For this review, take the finished solid that the model builds, in its own axes (mm). A direction names the side the tool comes from. Round coordinates to 2 decimals unless told otherwise and drop trailing zeros. Order: outer loops, then holes, each group sorted by start corner. A loop starts at its lowest first (then second) coordinate and runs counter-clockwise, first axis right, second up. Notation, with made-up numbers: (13.25, 20.25) - (32.25, 20.25) arc R27 cw to (32.25, 48.25) - close; hole circle Ø9 at (16, -27). An arc over 180 degrees is marked (long way). One line per question, with ' | ' between items.
```python
from build123d import *

# Parameters (mm, degrees)
ESQUISSE1_W                             = 30
ESQUISSE1_H                             = 10
BOSS_EXTRU_1_DEPTH                      = 130.5
ESQUISSE2_W                             = 30
ESQUISSE2_H                             = 5
BOSS_EXTRU_2_DEPTH                      = 20
PER_AGE_POUR_CROUS_AUTO_BLOQUANTS_300_D = 4.7625


with BuildPart() as part:
    # Esquisse1 → Boss.-Extru.1 (new body)
    with BuildSketch(Plane.XY):
        with Locations((15, 5)):
            Rectangle(ESQUISSE1_W, ESQUISSE1_H)
    extrude(amount=BOSS_EXTRU_1_DEPTH)

    # Esquisse2 → Boss.-Extru.2 (add)
    with BuildSketch(Plane.XZ):
        with Locations((15, 2.5)):
            Rectangle(ESQUISSE2_W, ESQUISSE2_H)
        with Locations((15, 18)):
            Rectangle(ESQUISSE2_W, ESQUISSE2_H)
        with Locations((15, 128)):
            Rectangle(ESQUISSE2_W, ESQUISSE2_H)
        with Locations((15, 112.5)):
            Rectangle(ESQUISSE2_W, ESQUISSE2_H)
    extrude(amount=BOSS_EXTRU_2_DEPTH)

    # Perçage pour écrous auto-bloquants 300® #6 (SP)1 (through all)
    with Locations(Plane.XY.offset(130.5)):
        with Locations((14.302143115, -10.686909811)):
            Hole(PER_AGE_POUR_CROUS_AUTO_BLOQUANTS_300_D / 2)


solid = part.part
```
(1) We need section B-B on x = 19.75. State the section outline as (y, z) points, plus the area to 4 significant figures.
Output values:
outline: (-20, 0) - (10, 0) - (10, 130.5) - (-20, 130.5) - (-20, 125.5) - (0, 125.5) - (0, 115) - (-20, 115) - (-20, 110) - (0, 110) - (0, 20.5) - (-20, 20.5) - (-20, 15.5) - (0, 15.5) - (0, 5) - (-20, 5) - close | area: 1,705 mm^2
(2) Insertion check: pin 1 (3 mm diameter, centred on x = 14, z = 8, fed in from -Y). The pin has a flat end and moves straight along its axis. Give the tip position at first contact, or say it passes through.
Output values:
pin 1: y = 0
(3) For probe 1 along Z at (x, y) = (9.25, -17.5); probe 2 along X at (y, z) = (-11, 16); probe 3 along Y at (x, z) = (23.25, 74), list the stretches that pass through material, from the lowest coordinate up. Write a range as [from, to].
Output values:
probe 1: [0, 5], [15.5, 20.5], [110, 115], [125.5, 130.5] | probe 2: [0, 11.94], [16.66, 30] | probe 3: [0, 10]
(4) We need section C-C on z = 88. State the section outline as (x, y) points.
Output values:
outline: (0, 0) - (30, 0) - (30, 10) - (0, 10) - close
(5) We need section A-A on y = -14.5. State the section outline as (x, z) points, plus the area to 3 significant figures.
Output values:
outline: (0, 0) - (30, 0) - (30, 5) - (0, 5) - close; (0, 15.5) - (30, 15.5) - (30, 20.5) - (0, 20.5) - close; (0, 110) - (30, 110) - (30, 115) - (0, 115) - close; (0, 125.5) - (30, 125.5) - (30, 130.5) - (0, 130.5) - close | area: 600 mm^2
(6) For faces 1 (the flat face through (15, 0, 120)), 2 (the flat face through (15, -20, 128)), list the 3-axis set-ups (+Z, -Z, +X, -X, +Y, -Y) from which the entire face can be reached by the end or side of a thin tool; tool diameter is ignored.
Output values:
face 1: +X, -X, -Y | face 2: +Z, -Z, +X, -X, -Y
(7) Mouldability with a two-part tool opening along Z and no side actions: class faces 3 (the flat face through (15, 0, 10)), 4 (the cylindrical face through (13.02, -8.68, 17.97)), 5 (the flat face through (15, -5, 0)) as released by +Z, released by -Z, zero draft, split by the parting line, or undercut.
Output values:
face 3: undercut | face 4: zero draft | face 5: released by -Z
